For this review, take the finished solid that the model builds, in its own axes (mm). Face numbers are marked on the shaded views. A direction names the side the tool comes from. Coordinates: 2 decimals unless noted, no trailing zeros. Order: outer loops, then holes, each group sorted by start corner. A loop starts at its lowest first (then second) coordinate and runs counter-clockwise, first axis right, second up. Notation, with made-up numbers: (-26.75, 31) -> (30.25, 31) arc R24 ccw to (30.25, 47) -> close; hole circle Ø3 at (62, -35). An arc over 180 degrees is marked (long way). Answer as a JSON object with one key per item and string values. Group by question number.
1) Add section C-C, the plane z = -0.25. Write out the cut boundary in (x, y).
2) Add section B-B, the plane y = 8.4. Write out the cut boundary in (x, z), then the cut area to 3 significant figures.
3) For pin 1 (0.6 mm diameter, centred on y = 17, z = -2.5, fed in from +X); pin 2 (2.5 mm diameter, centred on x = 13, y = 8.5, fed in from -Z), all flat-tipped, find the tip position at first contact; note any pin that passes through.
4) Add section A-A, the plane x = 8.7. Write out the cut boundary in (y, z), then the cut area to 3 significant figures.
5) Machinability: for the marked faces 1, 2, 3 and 4, which of the approach directions +Z, -Z, +X, -X, +Y, -Y give a long, thin tool a straight path to every point of the face, cutting with its end or side? Answer none if there is none.
6) Add section D-D, the plane y = 12.5. Write out the cut boundary in (x, z).
7) Wall thickness on L1, parallel to Y at x = 8.7, z = -2.4; L2, parallel to Y at x = 4, z = -2.25; L3, parallel to X at y = 16.5, z = 3: over which ranges is each line inside the solid? List them lowest first.
from build123d import *

# Parameters (mm, degrees)
SKETCH1_R                = 1.15
BOSS_EXTRUDE1_DEPTH      = 3.5
BOSS_EXTRUDE1_DEPTH_BACK = 3.5
SKETCH1_3_W              = 5
SKETCH1_3_H              = 20
BOSS_EXTRUDE2_DEPTH      = 1.5
BOSS_EXTRUDE2_DEPTH_BACK = 1.5


with BuildPart() as part:
    # Sketch1 → Boss-Extrude1 (new body, two sides)
    with BuildSketch(Plane.XY) as boss_extrude1_sk:
        Polygon((1, 0), (1, 3), (11, 3), (11, 23), (0, 23), (0, 0), align=None)
        with Locations((8.7, 8.4)):
            Circle(SKETCH1_R, mode=Mode.SUBTRACT)
        with Locations((8.7, 18)):
            Circle(SKETCH1_R, mode=Mode.SUBTRACT)
    extrude(amount=BOSS_EXTRUDE1_DEPTH)
    extrude(boss_extrude1_sk.sketch, amount=-BOSS_EXTRUDE1_DEPTH_BACK)

    # Sketch1_3 → Boss-Extrude2 (add, two sides)
    with BuildSketch(Plane.XY) as boss_extrude2_sk:
        with Locations((13.5, 13)):
            Rectangle(SKETCH1_3_W, SKETCH1_3_H)
    extrude(amount=BOSS_EXTRUDE2_DEPTH)
    extrude(boss_extrude2_sk.sketch, amount=-BOSS_EXTRUDE2_DEPTH_BACK)


solid = part.part
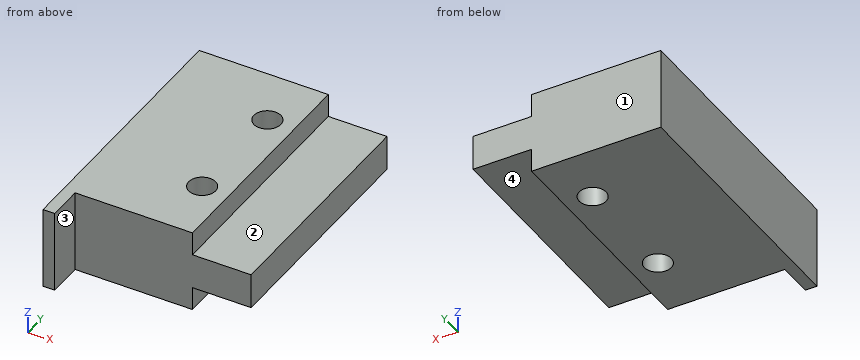
Output values:
{
 "1": {"outline": "(0, 0) -> (1, 0) -> (1, 3) -> (16, 3) -> (16, 23) -> (0, 23) -> close; hole circle Ø2.3 at (8.7, 8.4); hole circle Ø2.3 at (8.7, 18)"},
 "2": {"outline": "(0, -3.5) -> (7.55, -3.5) -> (7.55, 3.5) -> (0, 3.5) -> close; (9.85, -3.5) -> (11, -3.5) -> (11, -1.5) -> (16, -1.5) -> (16, 1.5) -> (11, 1.5) -> (11, 3.5) -> (9.85, 3.5) -> close", "area": "75.9 mm²"},
 "3": {"pin 1": "stops at x = 11", "pin 2": "stops at z = -1.5"},
 "4": {"outline": "(3, -3.5) -> (7.25, -3.5) -> (7.25, 3.5) -> (3, 3.5) -> close; (9.55, -3.5) -> (16.85, -3.5) -> (16.85, 3.5) -> (9.55, 3.5) -> close; (19.15, -3.5) -> (23, -3.5) -> (23, 3.5) -> (19.15, 3.5) -> close", "area": "108 mm²"},
 "5": {"face 1": "+Z, -Z, +X, -X, +Y", "face 2": "+Z, +X, +Y, -Y", "face 3": "+Z, -Z, +X, -Y", "face 4": "-Z, +X, +Y, -Y"},
 "6": {"outline": "(0, -3.5) -> (11, -3.5) -> (11, -1.5) -> (16, -1.5) -> (16, 1.5) -> (11, 1.5) -> (11, 3.5) -> (0, 3.5) -> close"},
 "7": {"L1": "y = 3 to 7.25, 9.55 to 16.85, 19.15 to 23", "L2": "y = 3 to 23", "L3": "x = 0 to 11"}
}
